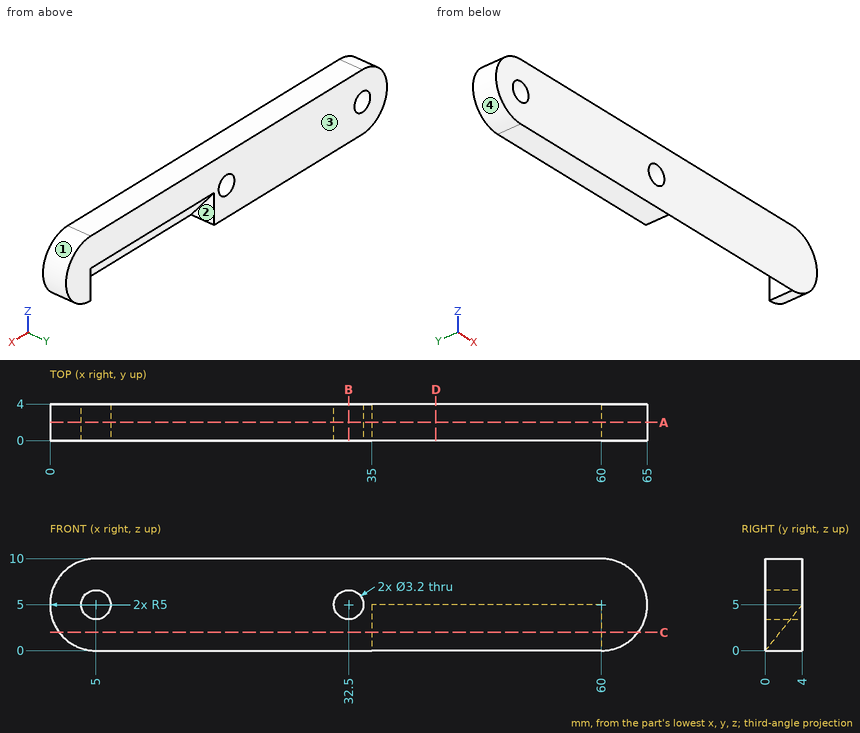
Answer from the drawing. Dimensions are ordinates in mm from the lowest x, y and z of the part. Coordinates: 2 decimals unless noted, no trailing zeros. Order: outer loops, then holes, each group sorted by start corner. A loop starts at its lowest first (then second) coordinate and runs counter-clockwise, first axis right, second up. Notation, with made-up numbers: (-39.5, 76.25) - (15.5, 76.25) arc R30 cw to (15.5, 105.25) - close; hole circle Ø11 at (-12, -10.75). An arc over 180 degrees is marked (long way). Answer as a JSON object with one key per item and string values. Group by question number.
Item 1: Section C-C (z = 2) is taken. Give the vertices of the cut face in (x, y), plus the area to 3 significant figures.
Item 2: Section D-D (x = 42) is taken. Give the vertices of the cut face in (y, z), plus the area to 3 significant figures.
Item 3: The mould has two halves that part along X. Classify the marked faces 1, 2, 3 and 4: +X half, -X half, draft (parallel to the pull), parting line (faces both ways), or undercut.
Item 4: Section B-B (x = 32.5) is taken. Give the vertices of the cut face in (y, z).
Item 5: Consider probe 1 along X at (y, z) = (2.55, 5); probe 2 along Z at (x, y) = (32.5, 2.7); probe 3 along X at (y, z) = (1.7, 5.75). Determine where each line is inside the solid, lowest interval first. Write a range as from..to.
Item 6: Flat-ended cylindrical pins translate along their axes: P1, Ø2, axis at y = 2, z = 3.5, coming from the -X side; P2, Ø1.5, axis at x = 40, y = 1.5, coming from the -Z side; P3, Ø1.2, axis at y = 3, z = 2, coming from the +X side; P4, Ø2.5, axis at x = 32.5, z = 5, coming from the -Y side. Find the tip coordinate at first contact, or state that the pin passes through.
Item 7: Section A-A (y = 2) is taken. Give the vertices of the cut face in (x, z).
Results are:
{
 "1": {"outline": "(1, 0) - (64, 0) - (64, 4) - (60, 4) - (60, 1.6) - (35, 1.6) - (35, 4) - (1, 4) - close", "area": "192 mm^2"},
 "2": {"outline": "(0, 0) - (4, 5) - (4, 10) - (0, 10) - close", "area": "30.0 mm^2"},
 "3": {"face 1": "+X half", "face 2": "undercut", "face 3": "draft", "face 4": "-X half"},
 "4": {"outline": "(0, 0) - (4, 0) - (4, 3.4) - (0, 3.4) - close; (0, 6.6) - (4, 6.6) - (4, 10) - (0, 10) - close"},
 "5": {"probe 1": "x = 0..3.4, 6.6..30.9, 34.1..65", "probe 2": "z = 0..3.4, 6.6..10", "probe 3": "x = 0.06..3.59, 6.41..31.09, 33.91..64.94"},
 "6": {"P1": "stops at x = 0.03", "P2": "stops at z = 0.94", "P3": "stops at x = 64.39", "P4": "passes through"},
 "7": {"outline": "(5, 0) - (35, 0) - (35, 2.5) - (60, 2.5) - (60, 0) arc R5 ccw to (60, 10) - (5, 10) arc R5 ccw to start; hole circle Ø3.2 at (5, 5); hole circle Ø3.2 at (32.5, 5)"}
}
